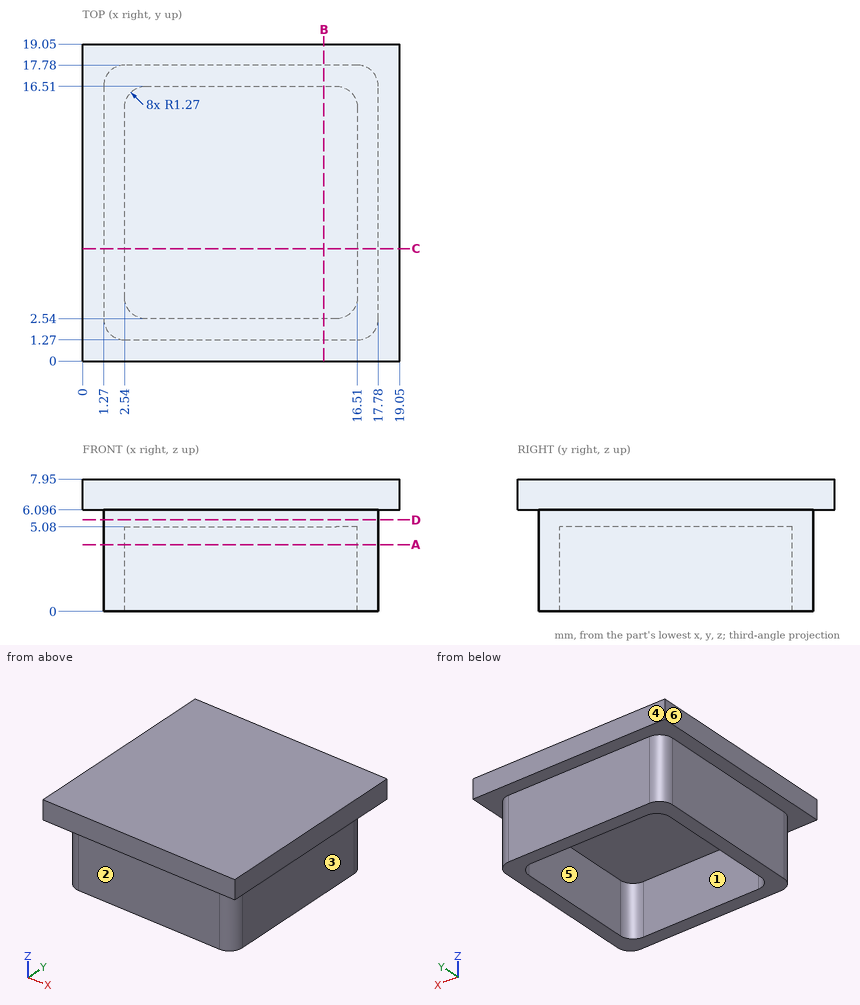
The figure shows three views and two pictorial views of one solid part (mm, origin at its lowest corner). Answer the questions. A direction names the side the tool comes from. Give positions to 0.01 mm unless a question says otherwise; leave off trailing zeros. Write each loop counter-clockwise with the first axis right and the second up, starting at its lowest first coordinate (ties: lowest second). Pieces come first, ordered by that corner, then holes.
Q1. The part is cut by section B-B on x = 14.5. Give the vertices of the cut face in (y, z), and give its area (3 significant figures).
Answer:
outline: (0, 6.1) - (1.27, 6.1) - (1.27, 0) - (2.54, 0) - (2.54, 5.08) - (16.51, 5.08) - (16.51, 0) - (17.78, 0) - (17.78, 6.1) - (19.05, 6.1) - (19.05, 7.95) - (0, 7.95) - close
area: 65.0 mm2
Q2. The part is cut by section A-A on z = 4. Give the vertices of the cut face in (x, y).
Answer:
outline: (1.27, 2.54) arc R1.27 ccw to (2.54, 1.27) - (16.51, 1.27) arc R1.27 ccw to (17.78, 2.54) - (17.78, 16.51) arc R1.27 ccw to (16.51, 17.78) - (2.54, 17.78) arc R1.27 ccw to (1.27, 16.51) - close; hole (2.54, 3.81) arc R1.27 ccw to (3.81, 2.54) - (15.24, 2.54) arc R1.27 ccw to (16.51, 3.81) - (16.51, 15.24) arc R1.27 ccw to (15.24, 16.51) - (3.81, 16.51) arc R1.27 ccw to (2.54, 15.24) - close
Q3. Straight lines are drawn through the part: L1, parallel to X at y = 14.5, z = 1; L2, parallel to Z at x = 13.75, y = 10.5. For each, find the intervals that lie inside material, in ascending order.
Answer:
L1: x = 1.27 to 2.54, 16.51 to 17.78
L2: z = 5.08 to 7.95
Q4. The part is cut by section D-D on z = 5.5. Give the vertices of the cut face in (x, y).
Answer:
outline: (1.27, 2.54) arc R1.27 ccw to (2.54, 1.27) - (16.51, 1.27) arc R1.27 ccw to (17.78, 2.54) - (17.78, 16.51) arc R1.27 ccw to (16.51, 17.78) - (2.54, 17.78) arc R1.27 ccw to (1.27, 16.51) - close
Q5. Given pin 1 (1.5 mm diameter, centred on y = 16, z = 5, fed in from +X); pin 2 (3 mm diameter, centred on y = 8.5, z = 2.5, fed in from -X); pin 3 (1 mm diameter, centred on y = 4.5, z = 6, fed in from -X); pin 4 (1.8 mm diameter, centred on x = 13, z = 4, fed in from -Y), each flat-ended and moving along its own axis, determine where each tip first touches the part or whether it passes through.
Answer:
pin 1: stops at x = 17.78
pin 2: stops at x = 1.27
pin 3: stops at x = 0
pin 4: stops at y = 1.27
Q6. A tool of negligible diameter and unlimited length cuts with its end or side. For the marked faces 1, 2 and 3, from which of +Z, -Z, +X, -X, +Y, -Y can it reach the whole face along a straight path? Write none if from no direction.
Answer:
face 1: -Z
face 2: -Z, +X, -X, -Y
face 3: -Z, +X, +Y, -Y
Q7. For a pull along Y with two mould halves and no side action, classify the marked faces 4, 5 and 6 as released by +Y, released by -Y, zero draft, split by the parting line, or undercut.
Answer:
face 4: released by +Y
face 5: undercut
face 6: zero draft
